Design review of the part built by this model. Coordinates are the model's own, in mm. Face numbers are marked on the shaded views. A direction names the side the tool comes from. Coordinates: 2 decimals unless noted, no trailing zeros. Write each loop counter-clockwise with the first axis right and the second up, starting at its lowest first coordinate (ties: lowest second). Pieces come first, ordered by that corner, then holes. Notation, with made-up numbers: M -23.5,-38 L -5.5,-38 A23 ccw -5.5,-19 Z; hole C 73.25,44 d5. An arc over 180 degrees is marked long. Write item = value, one per line.
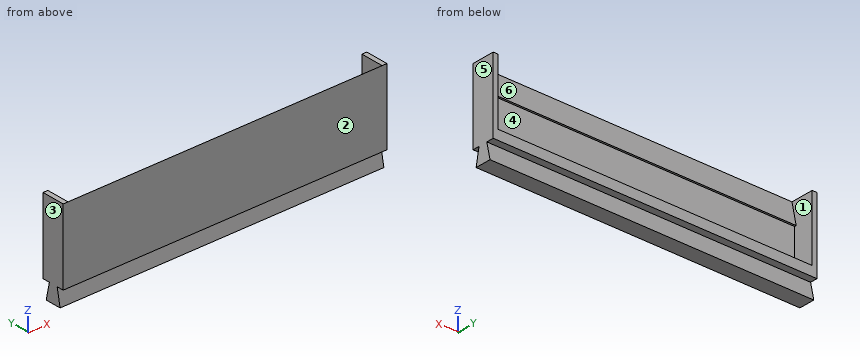
```python
from build123d import *

# Parameters (mm, degrees)
SKETCH1_W           = 163
SKETCH1_H           = 38.8
BOSS_EXTRUDE1_DEPTH = 2.5
CUT_EXTRUDE1_DEPTH  = 168
SKETCH4_W           = 27.063305406
SKETCH4_H           = 1
CUT_EXTRUDE2_DEPTH  = 168
SKETCH5_W           = 163
SKETCH5_H           = 5
BOSS_EXTRUDE2_DEPTH = 10.5
SKETCH6_W           = 38.8
SKETCH6_H           = 12
BOSS_EXTRUDE3_DEPTH = 2.5
SKETCH7_W           = 38.8
SKETCH7_H           = 12
BOSS_EXTRUDE4_DEPTH = 2.5
SKETCH8_W           = 168
SKETCH8_H           = 12
BOSS_EXTRUDE5_DEPTH = 8.8
SKETCH9_W           = 8.8
SKETCH9_H           = 1.9
SKETCH9_W_2         = 9
SKETCH9_H_2         = 1.8
CUT_EXTRUDE3_DEPTH  = 176.025026782


with BuildPart() as part:
    # Sketch1 → Boss-Extrude1 (new body)
    with BuildSketch(Plane(origin=(0, 0, 0), x_dir=(1, 0, 0), z_dir=(0, 1, 0))):
        with Locations((81.5, 19.4)):
            Rectangle(SKETCH1_W, SKETCH1_H)
    extrude(amount=BOSS_EXTRUDE1_DEPTH)

    # Sketch3 → Cut-Extrude1 (cut)
    with BuildSketch(Plane(origin=(163, 0, 0), x_dir=(0, 0, -1), z_dir=(1, 0, 0))):
        Polygon((0, 0), (11.736694594, 2.5), (0, 2.5), align=None)
    extrude(amount=-CUT_EXTRUDE1_DEPTH, mode=Mode.SUBTRACT)

    # Sketch4 → Cut-Extrude2 (cut)
    with BuildSketch(Plane(origin=(163, 0, 0), x_dir=(0, 0, -1), z_dir=(1, 0, 0))):
        with Locations((25.268347297, 2)):
            Rectangle(SKETCH4_W, SKETCH4_H)
    extrude(amount=-CUT_EXTRUDE2_DEPTH, mode=Mode.SUBTRACT)

    # Sketch5 → Boss-Extrude2 (add)
    with BuildSketch(Plane(origin=(0, 1.5, 0), x_dir=(1, 0, 0), z_dir=(0, 1, 0))):
        with Locations((81.5, 36.3)):
            Rectangle(SKETCH5_W, SKETCH5_H)
    extrude(amount=BOSS_EXTRUDE2_DEPTH)

    # Sketch6 → Boss-Extrude3 (add)
    with BuildSketch(Plane.ZY):
        with Locations((-19.4, 6)):
            Rectangle(SKETCH6_W, SKETCH6_H)
    extrude(amount=BOSS_EXTRUDE3_DEPTH)

    # Sketch7 → Boss-Extrude4 (add)
    with BuildSketch(Plane(origin=(163, 0, 0), x_dir=(0, 0, -1), z_dir=(1, 0, 0))):
        with Locations((19.4, 6)):
            Rectangle(SKETCH7_W, SKETCH7_H)
    extrude(amount=BOSS_EXTRUDE4_DEPTH)

    # Sketch8 → Boss-Extrude5 (add)
    with BuildSketch(Plane(origin=(0, 0, -38.8), x_dir=(-1, 0, 0), z_dir=(0, 0, -1))):
        with Locations((-81.5, 6)):
            Rectangle(SKETCH8_W, SKETCH8_H)
    extrude(amount=BOSS_EXTRUDE5_DEPTH)

    # Sketch9 → Cut-Extrude3 (cut, through all)
    with BuildSketch(Plane(origin=(165.5, 0, 0), x_dir=(0, 0, -1), z_dir=(1, 0, 0))):
        with Locations((43.2, 11.05)):
            Rectangle(SKETCH9_W, SKETCH9_H)
        Polygon((47.8, 1.8), (38.8, 3.6), (38.8, 1.8), align=None)
        Polygon((47.6, 10.1), (38.8, 10.1), (38.8, 8.2), align=None)
        with Locations((43.3, 0.9)):
            Rectangle(SKETCH9_W_2, SKETCH9_H_2)
    extrude(amount=-CUT_EXTRUDE3_DEPTH, mode=Mode.SUBTRACT)


solid = part.part
```
Q1. The part is to be moulded in two halves that separate along X. For the marked faces 1, 2 and 3, say which applies: +X half, -X half, draft (parallel to the pull), parting line (faces both ways), or undercut.
Check result:
face_1 = undercut
face_2 = draft
face_3 = -X half
Q2. For P1, Ø6.5, axis at x = 82.5, z = -18, coming from the +Y side; P2, Ø1.1, axis at x = 73.5, y = 1, coming from the -Z side; P3, Ø4, axis at x = 74.5, y = 7.5, coming from the +Z side, all flat-tipped, find the tip position at first contact; note any pin that passes through.
Check result:
P1 = 1.5
P2 = -38.8
P3 = -33.8
Q3. Consider section C-C, the plane z = -23.5. State the section outline as (x, y) points, and give its area (4 significant figures).
Check result:
outline = M -2.5,0 L 165.5,0 L 165.5,12 L 163,12 L 163,1.5 L 0,1.5 L 0,12 L -2.5,12 Z
area = 304.5 mm²
Q4. Consider section B-B, the plane y = 5.75. State the section outline as (x, z) points.
Check result:
outline = M -2.5,-47.6 L 165.5,-47.6 L 165.5,0 L 163,0 L 163,-33.8 L 0,-33.8 L 0,0 L -2.5,0 Z
Q5. Consider section A-A, the plane x = 155. State the section outline as (y, z) points, and give its area (3 significant figures).
Check result:
outline = M 0,-38.8 L 3.6,-38.8 L 1.84,-47.6 L 10.1,-47.6 L 8.2,-38.8 L 12,-38.8 L 12,-33.8 L 1.5,-33.8 L 1.5,-11.74 L 2.5,-11.74 L 0,0 Z
area = 164 mm²
Q6. Consider section D-D, the plane z = -43.5. State the section outline as (x, y) points.
Check result:
outline = M -2.5,2.66 L 165.5,2.66 L 165.5,9.21 L -2.5,9.21 Z
Q7. Wall thickness on line 1 (X direction, y = 3.5, z = -27); line 2 (Z direction, x = 41.5, y = 4.25); line 3 (Z direction, x = 62, y = 11.75): over which ranges is each line inside the solid? List them lowest first.
Check result:
line_1 = -2.5 to 0, 163 to 165.5
line_2 = -47.6 to -33.8
line_3 = -38.8 to -33.8
Q8. Machinability: for the marked faces 4, 5 and 6, which of the approach directions +Z, -Z, +X, -X, +Y, -Y give a long, thin tool a straight path to every point of the face, cutting with its end or side? Answer none if there is none.
Check result:
face_4 = +Y
face_5 = +Z, -Z, +X, +Y, -Y
face_6 = +Z, +Y
